Autodesk Inventor part; units mm, degrees
ref_plane "YZ Plane" through (0, 0, 0) normal (1, 0, 0) x (0, 1, 0)
ref_plane "XZ Plane" through (0, 0, 0) normal (0, 1, 0) x (-1, 0, 0)
ref_plane "XY Plane" through (0, 0, 0) normal (0, 0, 1) x (1, 0, 0)
sketch "Sketch2" plane through (0, 0, 0) normal (0, 1, 0) x (-1, 0, 0)
  line L0 (0, 0) -> (-220, 0)
  line L1 (-220, 0) -> (-220, -180)
  line L2 (-220, -180) -> (0, -180)
  line L3 (0, -180) -> (0, 0)
  dimension "d0" = 220
  dimension "d1" = 180
extrude "Extrusion1" add sketch "Sketch2" along normal blind 20
sketch "Sketch3" plane through (0, 20, 0) normal (0, 1, 0) x (1, 0, 0)
  line L0 (0, 20) -> (0, 160)
  line L1 (0, 90) -> (46.5, 90)
  line L2 (46.5, 90) -> (173.5, 90)
  line L3 (173.5, 90) -> (173.5, 109)
  line L4 (173.5, 109) -> (173.5, 71)
  line L5 (173.5, 71) -> (46.5, 71)
  line L6 (46.5, 71) -> (46.5, 109)
  line L7 (46.5, 109) -> (173.5, 109)
  line L8 (0, 0) -> (220, 0)
  line L9 (220, 0) -> (220, 180)
  line L10 (220, 180) -> (0, 180)
  line L11 (0, 180) -> (0, 0)
  dimension "d4" = 46.5
  dimension "d5" = 127
  dimension "d6" = 19
  dimension "d7" = 38
  dimension "d11" = 71
extrude "Extrusion2" cut sketch "Sketch3" against normal blind 10 contours L6 L7 L3 L2 | L2 L4 L5 L6
fillet "Fillet1" radius 20 4 edges at (0, 10, -180) (0, 10, 0) (220, 10, 0) (220, 10, -180)
fillet "Fillet2" radius 12 4 edges at (46.5, 15, -109) (173.5, 15, -109) (46.5, 15, -71) (173.5, 15, -71)
sketch "Sketch5" plane through (0, 0, 0) normal (0, -1, 0) x (1, 0, 0)
  line L0 (110, -90) -> (58.5, -90) construction
  line L1 (110, -90) -> (161.5, -90) construction
  line L2 (58.5, -90) -> (58.5, -97) construction
  line L3 (58.5, -97) -> (58.5, -83) construction
  line L4 (58.5, -83) -> (161.5, -83) construction
  line L5 (161.5, -83) -> (161.5, -97) construction
  circle A0 centre (58.5, -97) radius 2.5
  circle A1 centre (58.5, -83) radius 2.5
  circle A2 centre (161.5, -83) radius 2.5
  circle A3 centre (161.5, -94.5) radius 2.5
  line L6 (20, 0) -> (200, 0)
  arc A4 (200, -180) -> (220, -160) centre (200, -160) ccw
  line L7 (220, -20) -> (220, -160)
  arc A5 (220, -20) -> (200, 0) centre (200, -20) ccw
  line L8 (20, 0) -> (200, 0)
  arc A6 (20, 0) -> (0, -20) centre (20, -20) ccw
  line L9 (0, -160) -> (0, -20)
  arc A7 (0, -160) -> (20, -180) centre (20, -160) ccw
  line L10 (200, -180) -> (20, -180)
  point P0 (0, 0)
  point P1 (110, -90)
  dimension "d38" = 51.5
  dimension "d39" = 51.5
  dimension "d40" = 7
  dimension "d41" = 14
  dimension "d42" = 5
  dimension "d43" = 5
  dimension "d44" = 5
  dimension "d45" = 5
  dimension "d46" = 103
  dimension "d47" = 51.5
  dimension "d48" = 0
  dimension "d49" = 11.5
  dimension "d50" = 14
  dimension "d51" = 58.5
  dimension "d52" = 83
extrude "Extrusion4" cut sketch "Sketch5" against normal through all contours A0 | A1 | A2 | A3
properties part number "reverse gear stand"
The listing builds one solid part. Answer for the finished solid, in the listing's coordinates (mm). A direction names the side the tool comes from. Give positions to 0.01 mm unless a question says otherwise; leave off trailing zeros. Order: outer loops, then holes, each group sorted by start corner. A loop starts at its lowest first (then second) coordinate and runs counter-clockwise, first axis right, second up. Notation, with made-up numbers: (13, -13) -> (58, -13) arc R30 ccw to (58, 11) -> close; hole circle Ø8 at (1.5, 72). An arc over 180 degrees is marked (long way). Put each result on its own line as item: value.
Item 1: A cutting plane is placed at B-B on y = 14.25. Give the vertices of the cut face in (x, z).
Established:
outline: (0, -160) arc R20 ccw to (20, -180) -> (200, -180) arc R20 ccw to (220, -160) -> (220, -20) arc R20 ccw to (200, 0) -> (20, 0) arc R20 ccw to (0, -20) -> close; hole (46.5, -97) arc R12 ccw to (58.5, -109) -> (161.5, -109) arc R12 ccw to (173.5, -97) -> (173.5, -83) arc R12 ccw to (161.5, -71) -> (58.5, -71) arc R12 ccw to (46.5, -83) -> close
Item 2: For faces 1 (the face through (111, 15, -71)), 2 (the face through (111, 10, -180)), determine the directions among +Z, -Z, +X, -X, +Y, -Y from which every point of the face is accessible in a straight line to the end or side of a thin tool.
Established:
face 1: +Y
face 2: -Z, +X, -X, +Y, -Y
Item 3: A cutting plane is placed at A-A on x = 68. Give the vertices of the cut face in (y, z).
Established:
outline: (0, -180) -> (20, -180) -> (20, -109) -> (10, -109) -> (10, -71) -> (20, -71) -> (20, 0) -> (0, 0) -> close
Item 4: Straight lines are drawn through the part: line 1 (Z direction, x = 159, y = 19.25); line 2 (Z direction, x = 161.5, y = 4.75); line 3 (Y direction, x = 62, z = -95.5). For each, find the intervals that lie inside material, in ascending order.
Established:
line 1: z = -180 to -109, -71 to 0
line 2: z = -180 to -97, -92 to -85.5, -80.5 to 0
line 3: y = 0 to 10
Item 5: Given P1, Ø6, axis at x = 58.5, z = -83, coming from the +Y side, flat-ended and moving along its own axis, determine where the tip first touches the part or whether it passes through.
Established:
P1: stops at y = 10
Item 6: For a pull along X with two mould halves and no side action, classify faces 3 (the face through (0, 10, -91)), 4 (the face through (58.17, 4.93, -94.52)), 5 (the face through (109, 10, 0)) as released by +X, released by -X, zero draft, split by the parting line, or undercut.
Established:
face 3: released by -X
face 4: undercut
face 5: zero draft
